from build123d import *

# Parameters (mm, degrees)
BOSS_EXTRU_1_DEPTH         = 20
ESQUISSE2_R                = 1.5
ENL_V_MAT_EXTRU_1_DEPTH    = 2
R_P_TITION_LIN_AIRE1_COUNT = 2
R_P_TITION_LIN_AIRE1_PITCH = 10


with BuildPart() as part:
    # Esquisse1 → Boss.-Extru.1 (new body)
    with BuildSketch(Plane.XY):
        Polygon((1, 32.5), (1, 22.25), (7.5, 22.25), (7.5, 18.25), (5.5, 18.25), (3, 20.25), (5.5, 20.25), (5.5, 21.25), (1, 21.25), (1, 11.25), (5.5, 11.25), (5.5, 12.25), (3, 12.25), (5.5, 14.25), (7.5, 14.25), (7.5, 10.25), (1, 10.25), (1, 0), (0, 0), (0, 32.5), align=None)
    extrude(amount=BOSS_EXTRU_1_DEPTH)

    # Esquisse2 → Enlèv. mat.-Extru.1 (cut, through all)
    with BuildSketch(Plane(origin=(1, 0, 0), x_dir=(0, 0, -1), z_dir=(1, 0, 0))):
        with Locations((-15, 27.5)):
            Circle(ESQUISSE2_R)
        with Locations((-15, 5)):
            Circle(ESQUISSE2_R)
    enl_v_mat_extru_1 = extrude(amount=-ENL_V_MAT_EXTRU_1_DEPTH, mode=Mode.SUBTRACT)

    # Répétition linéaire1: Enlèv. mat.-Extru.1 ×2
    with Locations(*[(0, 0, -i * R_P_TITION_LIN_AIRE1_PITCH) for i in range(1, R_P_TITION_LIN_AIRE1_COUNT)]):
        add(enl_v_mat_extru_1, mode=Mode.SUBTRACT)


solid = part.part
Verification items for the finished model (mm, model axes). A direction names the side the tool comes from. Give positions to 0.01 mm unless a question says otherwise; leave off trailing zeros. Order: outer loops, then holes, each group sorted by start corner. A loop starts at its lowest first (then second) coordinate and runs counter-clockwise, first axis right, second up. Notation, with made-up numbers: M 78,74 L 123,74 A16 ccw 123,100 Z; hole C 60.5,-35 d7. An arc over 180 degrees is marked long. Use one line per item in the form item = value. Start each with the question number.
Q1. Access from +Z, -Z, +X, -X, +Y, -Y to the whole of each face (thin tool, end or side, straight path). Record for faces 5 (the flat face through (4, 10.25, 10)), 6 (the flat face through (4, 12.25, 10)), 7 (the cylindrical face through (0.51, 5.07, 6.5)), 8 (the flat face through (6, 14.25, 10)).
Q2. Mould release check, pull along Y, two halves, no side actions. Record for faces 1 (the cylindrical face through (0.507, 28.987, 5.195)), 2 (the flat face through (0.5, 0, 9.9)), 3 (the flat face through (0, 16, 10)), 4 (the flat face through (4, 20.25, 10)): +Y half, -Y half, draft (parallel to the pull), parting line (faces both ways), or undercut.
Q3. Section check B-B (y = 27.5). Enter the section's corners in (x, z).
Q4. Section check A-A (x = 4). Enter the section's corners in (y, z), then the cut area to 3 significant figures.
Q5. Section check C-C (x = 2.25). Enter the section's corners in (y, z), then the cut area to 3 significant figures.
Q6. Section check D-D (z = 5). Enter the section's corners in (x, y).
Q7. Go/stop test with flat-tipped pins: pin 1 Ø0.8 at (x, z) = (3.5, 6) entering from +Y; pin 2 Ø1.6 at (x, z) = (7, 8) entering from -Y; pin 3 Ø1.8 at (y, z) = (27.5, 15) entering from +X; pin 4 Ø8 at (y, z) = (6, 13) entering from +X. Record where each tip stops, or that it passes through.
Q8. Scan lines: line 1 along Y through (x, z) = (0.75, 15); line 2 along Y through (x, z) = (1.75, 8); line 3 along Y through (x, z) = (7.25, 4). Record each from-to range of solid material in increasing order. Write a range as [from, to].
Evaluation:
q1.face_5 = +Z, -Z, +X, -Y
q1.face_6 = +Z, -Z
q1.face_7 = +X, -X
q1.face_8 = +Z, -Z, +X
q2.face_1 = undercut
q2.face_2 = -Y half
q2.face_3 = draft
q2.face_4 = undercut
q3.outline = M 0,0 L 1,0 L 1,3.5 L 0,3.5 Z; M 0,6.5 L 1,6.5 L 1,13.5 L 0,13.5 Z; M 0,16.5 L 1,16.5 L 1,20 L 0,20 Z
q4.outline = M 10.25,0 L 11.25,0 L 11.25,20 L 10.25,20 Z; M 12.25,0 L 13.05,0 L 13.05,20 L 12.25,20 Z; M 19.45,0 L 20.25,0 L 20.25,20 L 19.45,20 Z; M 21.25,0 L 22.25,0 L 22.25,20 L 21.25,20 Z
q4.area = 72.0 mm2
q5.outline = M 10.25,0 L 11.25,0 L 11.25,20 L 10.25,20 Z; M 21.25,0 L 22.25,0 L 22.25,20 L 21.25,20 Z
q5.area = 40.0 mm2
q6.outline = M 0,0 L 1,0 L 1,3.5 L 0,3.5 Z; M 0,6.5 L 1,6.5 L 1,10.25 L 7.5,10.25 L 7.5,14.25 L 5.5,14.25 L 3,12.25 L 5.5,12.25 L 5.5,11.25 L 1,11.25 L 1,21.25 L 5.5,21.25 L 5.5,20.25 L 3,20.25 L 5.5,18.25 L 7.5,18.25 L 7.5,22.25 L 1,22.25 L 1,26 L 0,26 Z; M 0,29 L 1,29 L 1,32.5 L 0,32.5 Z
q7.pin_1 = 22.25
q7.pin_2 = 10.25
q7.pin_3 = through
q7.pin_4 = 1
q8.line_1 = [0, 3.5], [6.5, 26], [29, 32.5]
q8.line_2 = [10.25, 11.25], [21.25, 22.25]
q8.line_3 = [10.25, 14.25], [18.25, 22.25]
